Part model, mm, in its own coordinate system. Face numbers are marked on the shaded views. A direction names the side the tool comes from. Coordinates: 2 decimals unless noted, no trailing zeros. Loops run counter-clockwise (first coordinate to the right, second up) from the corner with the lowest first, then second, coordinate; pieces in that order, holes last.
```python
from build123d import *

# Parameters (mm, degrees)
BOSS_EXTRUDE1_DEPTH  = 40
M6_CLEARANCE_HOLE1_D = 6.6
M6_CLEARANCE_HOLE2_D = 6.6
FILLET1_R            = 1
FILLET2_R            = 0.5
CUT_EXTRUDE1_DEPTH   = 73.498275842


with BuildPart() as part:
    # Sketch1 → Boss-Extrude1 (new body)
    with BuildSketch(Plane.XY):
        Polygon((0, 0), (40, 0), (40, 6), (6, 6), (6, 50), (0, 50), align=None)
    extrude(amount=BOSS_EXTRUDE1_DEPTH)

    # M6 Clearance Hole1 (through all)
    with Locations(Plane(origin=(6, 0, 0), x_dir=(0, 0, -1), z_dir=(1, 0, 0))):
        with Locations((-20, 40), (-20, 20)):
            Hole(M6_CLEARANCE_HOLE1_D / 2)

    # M6 Clearance Hole2 (through all)
    with Locations(Plane(origin=(0, 0, 0), x_dir=(-1, 0, 0), z_dir=(0, -1, 0))):
        with Locations((-22.5, -32.5), (-22.5, -7.5)):
            Hole(M6_CLEARANCE_HOLE2_D / 2)

    # Fillet1
    fillet1_edges = [part.edges().sort_by_distance(p)[0] for p in [
        (6, 6, 20),
    ]]
    fillet(fillet1_edges, radius=FILLET1_R)

    # Fillet2
    fillet2_edges = [part.edges().sort_by_distance(p)[0] for p in [
        (0, 0, 20),
    ]]
    fillet(fillet2_edges, radius=FILLET2_R)

    # Sketch7 → Cut-Extrude1 (cut, through all)
    with BuildSketch(Plane(origin=(6, 0, 0), x_dir=(0, 0, -1), z_dir=(1, 0, 0))):
        with BuildLine():
            Line((-5, 50), (0, 50))
            Line((0, 50), (0, 15))
            ThreePointArc((0, 15), (-3.535533906, 16.464466094), (-5, 20))
            Line((-5, 20), (-5, 50))
        make_face()
        with BuildLine():
            Line((-35, 20), (-35, 50))
            Line((-35, 50), (-40, 50))
            Line((-40, 50), (-40, 15))
            ThreePointArc((-40, 15), (-36.464466094, 16.464466094), (-35, 20))
        make_face()
    extrude(amount=-CUT_EXTRUDE1_DEPTH, mode=Mode.SUBTRACT)


solid = part.part
```
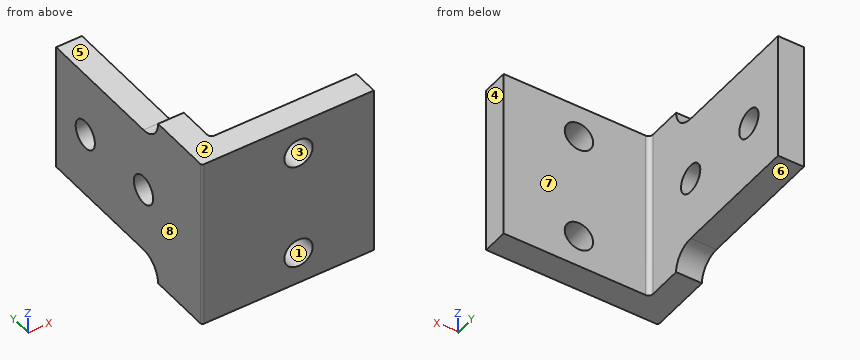
Q1. Tool access for the marked faces 5, 6, 7 and 8: list every direction of +Z, -Z, +X, -X, +Y, -Y with a clear straight run to the whole face (end or side of a thin tool).
Q2. Probe line 1 (Y direction, x = 2, z = 20); line 2 (Z direction, x = 22.5, y = 2.2); line 3 (Y direction, x = 31, z = 5). List the from-to ranges inside material, lowest first.
Q3. Saw through at C-C (x = 3.5). List the corners of the cut face in (y, z).
Q4. Drop flat-ended pins along their axis: P1, Ø5.5, axis at y = 20, z = 20, coming from the +X side; P2, Ø6, axis at y = 37.5, z = 34.5, coming from the +X side; P3, Ø5, axis at x = 3.5, y = 30, coming from the +Z side; P4, Ø6.5, axis at x = 4, y = 42, coming from the -Z side. Give the stop position or say it passes through.
Q5. Saw through at B-B (x = 22.5). List the corners of the cut face in (y, z), plus the area to 3 significant figures.
Q6. Saw through at D-D (z = 20). List the corners of the cut face in (x, y), plus the area to 3 significant figures.
Q7. Mould opens along X. For the marked faces 1, 2, 3 and 4 say: released by +X, released by -X, zero draft, split by the parting line, or undercut.
Q8. Saw through at A-A (z = 7.5). List the corners of the cut face in (x, y), plus the area to 3 significant figures.
Checked values:
1. face 5: +Z, +X, -X, +Y
1. face 6: -Z, +X, -X, +Y
1. face 7: +Z, -Z, +X, +Y
1. face 8: +Z, -Z, -X, +Y, -Y
2. line 1: y = 0 to 16.7, 23.3 to 36.7, 43.3 to 50
2. line 2: z = 0 to 4.2, 10.8 to 29.2, 35.8 to 40
2. line 3: y = 0 to 6
3. outline: (0, 0) - (15, 0) arc R5 cw to (20, 5) - (50, 5) - (50, 35) - (20, 35) arc R5 cw to (15, 40) - (0, 40) - close; hole circle Ø6.6 at (20, 20); hole circle Ø6.6 at (40, 20)
4. P1: passes through
4. P2: stops at x = 6
4. P3: stops at z = 35
4. P4: stops at z = 5
5. outline: (0, 0) - (6, 0) - (6, 4.2) - (0, 4.2) - close; (0, 10.8) - (6, 10.8) - (6, 29.2) - (0, 29.2) - close; (0, 35.8) - (6, 35.8) - (6, 40) - (0, 40) - close
5. area: 161 mm2
6. outline: (0, 0.5) arc R0.5 ccw to (0.5, 0) - (40, 0) - (40, 6) - (7, 6) arc R1 cw to (6, 7) - (6, 16.7) - (0, 16.7) - close; (0, 23.3) - (6, 23.3) - (6, 36.7) - (0, 36.7) - close; (0, 43.3) - (6, 43.3) - (6, 50) - (0, 50) - close
6. area: 425 mm2
7. face 1: undercut
7. face 2: zero draft
7. face 3: undercut
7. face 4: released by +X
8. outline: (0, 0.5) arc R0.5 ccw to (0.5, 0) - (19.2, 0) - (19.2, 6) - (7, 6) arc R1 cw to (6, 7) - (6, 50) - (0, 50) - close; (25.8, 0) - (40, 0) - (40, 6) - (25.8, 6) - close
8. area: 465 mm2
